from build123d import *

# Parameters (mm, degrees)
F0_R           = 44.7
F1_DEPTH       = 8
F0_R_2         = 52.7000017464
F2_DEPTH       = 20
F4_D           = 6.6
F4_CBORE_D     = 11.25
F4_CBORE_DEPTH = 6
F5_SIZE        = 2


with BuildPart() as f1:
    # F0 (on Top) → F1 (new body)
    with BuildSketch(Plane.XY):
        Circle(F0_R)
    extrude(amount=F1_DEPTH)

    # F0 (on Top) → F2 (join)
    with BuildSketch(Plane.XY):
        Circle(F0_R_2)
        Circle(F0_R, mode=Mode.SUBTRACT)
    extrude(amount=F2_DEPTH)

    # F4 (through all)
    with Locations(Plane.XY.offset(8)):
        with Locations((-30.4298021065, 0), (29.5701978935, 0)):
            CounterBoreHole(F4_D / 2, F4_CBORE_D / 2, F4_CBORE_DEPTH)

    # F5
    f5_edges = [f1.edges().sort_by_distance(p)[0] for p in [
        (-52.700002, 0, 0),
        (-52.700002, 0, 20),
        (-44.7, 0, 20),
    ]]
    chamfer(f5_edges, length=F5_SIZE)


solid = f1.part
Design review of the part built by this model. Coordinates are the model's own, in mm. A direction names the side the tool comes from. Coordinates: 2 decimals unless noted, no trailing zeros. Order: outer loops, then holes, each group sorted by start corner. A loop starts at its lowest first (then second) coordinate and runs counter-clockwise, first axis right, second up. Notation, with made-up numbers: (35.25, 78.5) -> (57.25, 78.5) arc R24 cw to (57.25, 99.5) -> close; hole circle Ø3 at (20, -17). An arc over 180 degrees is marked (long way). Use one line per item in the form item = value. Start each with the question number.
(1) The part is to be moulded in two halves that separate along Y. For faces 3 (the flat face through (-1, 1, 0)), 4 (the cylindrical face through (-5.82, 44.32, 12.93)), 5 (the cylindrical face through (26.52, -1.26, 0.99)), 6 (the cylindrical face through (-41.82, -32.07, 9.89)), say which applies: +Y half, -Y half, draft (parallel to the pull), parting line (faces both ways), or undercut.
(2) Add section C-C on z = 6. State the section outline as (x, y) points (3 decimals).
(3) Insertion check: pin 1 (4 mm diameter, centred on x = -30.43, y = 0, fed in from -Z); pin 2 (3.5 mm diameter, centred on x = -33, y = -1.5, fed in from +Z); pin 3 (1 mm diameter, centred on x = 28.5, z = 11, fed in from +Y); pin 4 (4 mm diameter, centred on y = 12.5, z = 15.5, fed in from +X). Each pin has a flat end and moves straight along its axis. Give the tip position at first contact, or say it passes through.
(4) Add section B-B on x = 0. State the section outline as (y, z) points.
(5) For faces 1 (the cylindrical face through (-33.577, 0.991, 0.986)), 2 (the cylindrical face through (34.935, 1.69, 5.042)), list the 3-axis set-ups (+Z, -Z, +X, -X, +Y, -Y) from which the entire face can be reached by the end or side of a thin tool; tool diameter is ignored.
(6) For probe 1 along Z at (x, y) = (-5.5, 41); probe 2 along X at (y, z) = (-41, 18.25); probe 3 along X at (y, z) = (-13, 13.75), list the stretches that pass through material, from the lowest coordinate up.
(7) Add section A-A on y = 0. Give the number of separate pieces and of enclosed holes in the cut face, plus the area to 3 significant figures.
Answer block:
q1.face_3 = draft
q1.face_4 = undercut
q1.face_5 = undercut
q1.face_6 = parting line
q2.outline = circle Ø105.4 at (0, 0); hole circle Ø11.25 at (-30.43, 0); hole circle Ø11.25 at (29.57, 0)
q3.pin_1 = through
q3.pin_2 = 2
q3.pin_3 = 44.65
q3.pin_4 = 51.64
q4.outline = (-52.7, 2) -> (-50.7, 0) -> (50.7, 0) -> (52.7, 2) -> (52.7, 18) -> (50.7, 20) -> (46.7, 20) -> (44.7, 18) -> (44.7, 8) -> (-44.7, 8) -> (-44.7, 18) -> (-46.7, 20) -> (-50.7, 20) -> (-52.7, 18) -> close
q5.face_1 = +Z, -Z
q5.face_2 = +Z
q6.probe_1 = 0 to 8
q6.probe_2 = -32.71 to -18.43, 18.43 to 32.71
q6.probe_3 = -51.07 to -42.77, 42.77 to 51.07
q7.separate_pieces = 3
q7.enclosed_holes = 0
q7.area = 862 mm²
